Geometry: final body of the model. Coordinates: model frame, mm. A direction names the side the tool comes from. Round coordinates to 2 decimals unless told otherwise and drop trailing zeros. Loops run counter-clockwise (first coordinate to the right, second up) from the corner with the lowest first, then second, coordinate; pieces in that order, holes last. Notation, with made-up numbers: (24, 77) - (49, 77) arc R13 cw to (49, 97) - close; hole circle Ø10 at (55.25, 9). An arc over 180 degrees is marked (long way). Return JSON: item names as keys, results as strings. Group by question number.
1. Section C-C on y = 0. Return loops of the section in (x, z) (3 decimals).
2. First-contact query: pin 1 Ø5 at (y, z) = (-33, 11) entering from +X (3 decimals); pin 2 Ø8 at (x, y) = (-6, 16) entering from -Z; pin 3 Ø1.6 at (x, z) = (23.5, 7.5) entering from -Y (3 decimals); pin 4 Ø5.5 at (x, y) = (14.5, 13.5) entering from +Z (3 decimals). Flat tips, straight axial feed; report the tip coordinate or a pass-through.
3. Section B-B on z = 21. Return loops of the section in (x, y) (3 decimals).
4. Set-up query: faces 1 (the face through (-22.225, 25, 19)), 2 (the face through (-11.967, -42.353, 7.826)), 3 (the face through (-27, 15.875, 27)), 4 (the face through (-28.62, 22.47, 24.53)). Return all of +Z, -Z, +X, -X, +Y, -Y with unobstructed straight access to the full face (end or side cutting, diameter ignored); none if empty.
5. Material intervals for probe 1 along X at (y, z) = (0, 6) (3 decimals); probe 2 along X at (y, z) = (25, 22.5) (3 decimals); probe 3 along Z at (x, y) = (-15.1, -38.1) (1 decimal), sorted ascending.
6. Section A-A on y = 25.4. Count the separate pieces of the cut face and the enclosed holes in it, and give its area (3 significant figures).
7. Section D-D on y = -24.5. Return loops of the section in (x, z) (1 decimal), and give its area (3 significant figures).
8. Draft query along Z for faces 5 (the face through (16, 14, 15.875)), 6 (the face through (-31.75, 17, 15)), 7 (the face through (-23.79, 22.47, 32.84)). Return one class per face: +Z half, -Z half, draft (parallel to the pull), parting line (faces both ways), or undercut.
from build123d import *

# Parameters (mm, degrees)
F0_R      = 12.7
F1_DEPTH  = 38.1
F2_W      = 69.85
F2_H      = 22.225
F3_DEPTH  = 63.501
F4_W      = 12.7
F4_H      = 29.490311
F5_DEPTH  = 88.951801
F6_R      = 3.96875
F6_R_2    = 3.175
F7_DEPTH  = 63.501
F8_R      = 6.35
F9_DEPTH  = 6.35
F10_R     = 6.35
F11_DEPTH = 6.35


with BuildPart() as f1:
    # F0 (on Top) → F1 (new body)
    with BuildSketch(Plane.XY):
        with BuildLine():
            ThreePointArc((-1.5875, -50.700391), (-12.7, -38.1), (-1.5875, -25.499609))
            Line((-1.5875, -25.499609), (-1.5875, -15.875))
            Line((-1.5875, -15.875), (1.5875, -15.875))
            Line((1.5875, -15.875), (1.5875, -25.499609))
            ThreePointArc((1.5875, -25.499609), (12.7, -38.1), (1.5875, -50.700391))
            Line((1.5875, -50.700391), (1.5875, -53.975))
            Line((1.5875, -53.975), (14.605, -53.975))
            ThreePointArc((14.605, -53.975), (15.503026, -53.603026), (15.875, -52.705))
            Line((15.875, -52.705), (15.875, -22.225))
            ThreePointArc((15.875, -22.225), (17.734872, -17.734872), (22.225, -15.875))
            Line((22.225, -15.875), (25.4, -15.875))
            ThreePointArc((25.4, -15.875), (29.890128, -14.015128), (31.75, -9.525))
            Line((31.75, -9.525), (31.75, 33.705801))
            ThreePointArc((31.75, 33.705801), (31.378026, 34.603826), (30.48, 34.975801))
            Line((30.48, 34.975801), (23.495, 34.975801))
            ThreePointArc((23.495, 34.975801), (22.596974, 34.603826), (22.225, 33.705801))
            Line((22.225, 33.705801), (22.225, 15.98998))
            ThreePointArc((22.225, 15.98998), (22.206202, 15.944598), (22.160821, 15.925801))
            Line((22.160821, 15.925801), (9.589179, 15.925801))
            ThreePointArc((9.589179, 15.925801), (9.543798, 15.944598), (9.525, 15.98998))
            Line((9.525, 15.98998), (9.525, 33.705801))
            ThreePointArc((9.525, 33.705801), (9.153026, 34.603826), (8.255, 34.975801))
            Line((8.255, 34.975801), (-8.255, 34.975801))
            ThreePointArc((-8.255, 34.975801), (-9.153026, 34.603826), (-9.525, 33.705801))
            Line((-9.525, 33.705801), (-9.525, 15.925801))
            Line((-9.525, 15.925801), (-22.225, 15.925801))
            Line((-22.225, 15.925801), (-22.225, 33.705801))
            ThreePointArc((-22.225, 33.705801), (-22.596974, 34.603826), (-23.495, 34.975801))
            Line((-23.495, 34.975801), (-30.48, 34.975801))
            ThreePointArc((-30.48, 34.975801), (-31.378026, 34.603826), (-31.75, 33.705801))
            Line((-31.75, 33.705801), (-31.75, -9.525))
            ThreePointArc((-31.75, -9.525), (-29.890128, -14.015128), (-25.4, -15.875))
            Line((-25.4, -15.875), (-22.225, -15.875))
            ThreePointArc((-22.225, -15.875), (-17.734872, -17.734872), (-15.875, -22.225))
            Line((-15.875, -22.225), (-15.875, -52.705))
            ThreePointArc((-15.875, -52.705), (-15.503026, -53.603026), (-14.605, -53.975))
            Line((-14.605, -53.975), (-1.5875, -53.975))
            Line((-1.5875, -53.975), (-1.5875, -50.700391))
        make_face()
        with Locations((-15.875, 0)):
            Circle(F0_R, mode=Mode.SUBTRACT)
        with Locations((15.875, 0)):
            Circle(F0_R, mode=Mode.SUBTRACT)
    extrude(amount=F1_DEPTH)

    # F2 (on face) → F3 (cut, through all)
    with BuildSketch(Plane.YZ.offset(31.75)):
        with Locations((-19.05, 26.9875)):
            Rectangle(F2_W, F2_H)
    extrude(amount=-F3_DEPTH, mode=Mode.SUBTRACT)

    # F4 (on face) → F5 (cut, through all)
    with BuildSketch(Plane(origin=(0, 34.975801, 0), x_dir=(-1, 0, 0), z_dir=(0, 1, 0))):
        with Locations((15.875, 30.620155)):
            Rectangle(F4_W, F4_H)
        with Locations((-15.875, 30.620155)):
            Rectangle(F4_W, F4_H)
    extrude(amount=-F5_DEPTH, mode=Mode.SUBTRACT)

    # F6 (on face) → F7 (cut, through all)
    with BuildSketch(Plane.YZ.offset(31.75)):
        with Locations((25.4, 30.1625)):
            Circle(F6_R)
        with Locations((-38.1, 7.9375)):
            Circle(F6_R_2)
    extrude(amount=-F7_DEPTH, mode=Mode.SUBTRACT)

    # F8 (on face) → F9 (cut)
    with BuildSketch(Plane.YZ.offset(31.75)):
        with Locations((25.4, 30.1625)):
            Circle(F8_R)
    extrude(amount=-F9_DEPTH, mode=Mode.SUBTRACT)

    # F10 (on face) → F11 (cut)
    with BuildSketch(Plane(origin=(-31.75, 0, 0), x_dir=(0, -1, 0), z_dir=(-1, 0, 0))):
        with Locations((-25.4, 30.1625)):
            Circle(F10_R)
    extrude(amount=-F11_DEPTH, mode=Mode.SUBTRACT)


solid = f1.part
Taken from the geometry:
{
 "1": {"outline": "(-31.75, 0) - (-28.575, 0) - (-28.575, 15.875) - (-31.75, 15.875) - close; (-3.175, 0) - (3.175, 0) - (3.175, 15.875) - (-3.175, 15.875) - close; (28.575, 0) - (31.75, 0) - (31.75, 15.875) - (28.575, 15.875) - close"},
 "2": {"pin 1": "x = 15.875", "pin 2": "z = 0", "pin 3": "y = -15.875", "pin 4": "z = 15.875"},
 "3": {"outline": "(-31.75, 15.875) - (-22.225, 15.875) - (-22.225, 33.706) arc R1.27 ccw to (-23.495, 34.976) - (-30.48, 34.976) arc R1.27 ccw to (-31.75, 33.706) - close; (-9.525, 15.875) - (9.525, 15.875) - (9.525, 33.706) arc R1.27 ccw to (8.255, 34.976) - (-8.255, 34.976) arc R1.27 ccw to (-9.525, 33.706) - close; (22.225, 15.875) - (31.75, 15.875) - (31.75, 33.706) arc R1.27 ccw to (30.48, 34.976) - (23.495, 34.976) arc R1.27 ccw to (22.225, 33.706) - close"},
 "4": {"face 1": "+Z, -Z, +Y", "face 2": "+Z, -Z", "face 3": "+Z, +X, -X, -Y", "face 4": "-X"},
 "5": {"probe 1": "-31.75 to -28.575, -3.175 to 3.175, 28.575 to 31.75", "probe 2": "-31.75 to -22.225, -9.525 to 9.525, 22.225 to 31.75", "probe 3": "0 to 4.8, 11.1 to 15.9"},
 "6": {"separate pieces": "6", "enclosed holes": "0", "area": "1,090 mm2"},
 "7": {"outline": "(-15.9, 0) - (-1.6, 0) - (-1.6, 15.9) - (-15.9, 15.9) - close; (1.6, 0) - (15.9, 0) - (15.9, 15.9) - (1.6, 15.9) - close", "area": "454 mm2"},
 "8": {"face 5": "+Z half", "face 6": "draft", "face 7": "undercut"}
}
